Check sheet for the drawn part. Datum: minimum x, y, z corner. Units: mm. Give positions to 0.01 mm unless a question says otherwise; leave off trailing zeros. Write each loop counter-clockwise with the first axis right and the second up, starting at its lowest first coordinate (ties: lowest second). Pieces come first, ordered by that corner, then holes. Notation, with made-up numbers: (27.25, -3.5) - (64.25, -3.5) arc R28 cw to (64.25, 32.5) - close; hole circle Ø9 at (4.25, 85). An arc over 180 degrees is marked (long way). Answer as a JSON object with one key per item and string values. Group by question number.
Item 1: Sectioned sample at B-B, the plane x = 5. Record the boundary of the cut face in (y, z).
Item 2: Scan lines: line 1 along Y through (x, z) = (5, 1.2); line 2 along X through (y, z) = (25, 1.5); line 3 along Y through (x, z) = (7, 1.7). Record each from-to range of solid material in increasing order. Write a range as [from, to].
Item 3: Sectioned sample at C-C, the plane z = 1.55. Record the boundary of the cut face in (x, y).
Item 4: Sectioned sample at A-A, the plane y = 5. Record the boundary of the cut face in (x, z), and give its area (3 significant figures).
Item 5: Draft check along X on the marked faces 1, 2, 3 and 4. Enter one of: +X half, -X half, draft (parallel to the pull), parting line (faces both ways), or undercut.
Item 6: Sectioned sample at D-D, the plane x = 3.25. Record the boundary of the cut face in (y, z).
Item 7: Go/stop test with flat-tipped pins: pin 1 (2 mm diameter, centred on x = 8, y = 10.5, fed in from -Z); pin 2 (5.5 mm diameter, centred on x = 5, y = 25, fed in from -Z). Record where each tip stops, or that it passes through.
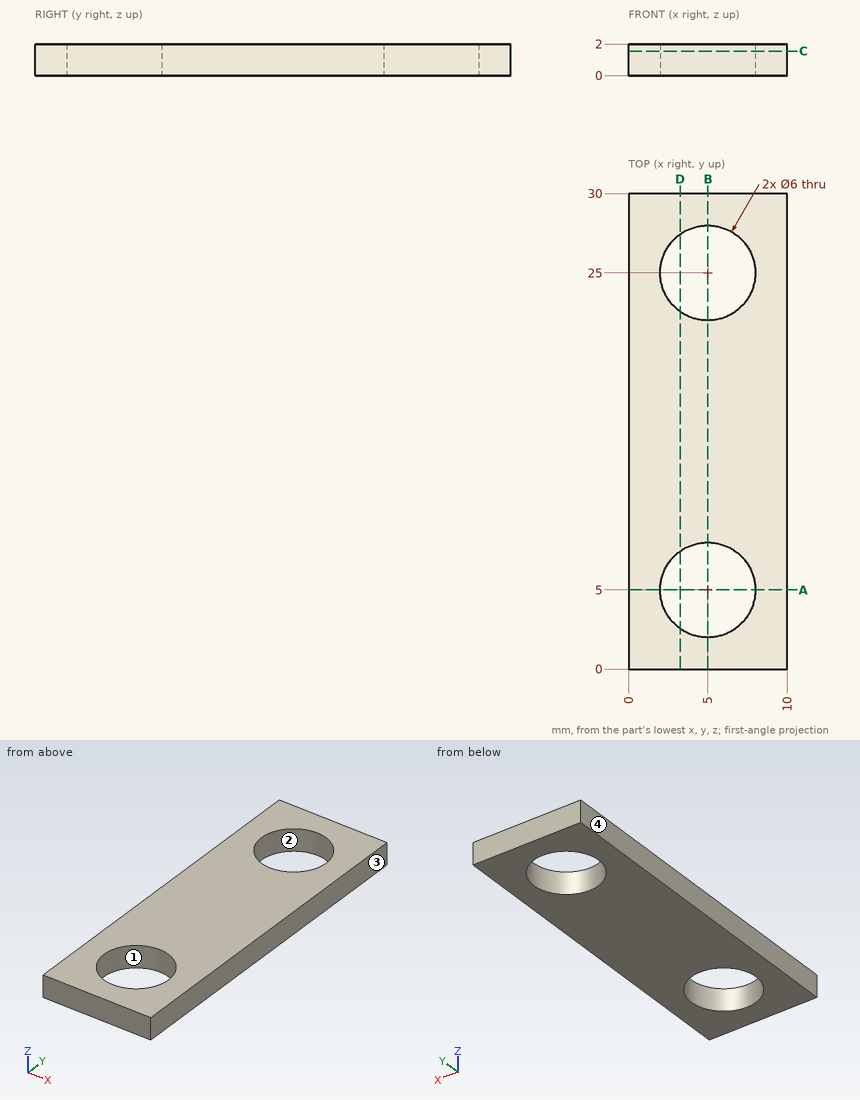
Geometry check:
{
 "1": {"outline": "(0, 0) - (2, 0) - (2, 2) - (0, 2) - close; (8, 0) - (22, 0) - (22, 2) - (8, 2) - close; (28, 0) - (30, 0) - (30, 2) - (28, 2) - close"},
 "2": {"line 1": "[0, 2], [8, 22], [28, 30]", "line 2": "[0, 2], [8, 10]", "line 3": "[0, 2.76], [7.24, 22.76], [27.24, 30]"},
 "3": {"outline": "(0, 0) - (10, 0) - (10, 30) - (0, 30) - close; hole circle Ø6 at (5, 5); hole circle Ø6 at (5, 25)"},
 "4": {"outline": "(0, 0) - (2, 0) - (2, 2) - (0, 2) - close; (8, 0) - (10, 0) - (10, 2) - (8, 2) - close", "area": "8.00 mm^2"},
 "5": {"face 1": "undercut", "face 2": "undercut", "face 3": "+X half", "face 4": "-X half"},
 "6": {"outline": "(0, 0) - (2.56, 0) - (2.56, 2) - (0, 2) - close; (7.44, 0) - (22.56, 0) - (22.56, 2) - (7.44, 2) - close; (27.44, 0) - (30, 0) - (30, 2) - (27.44, 2) - close"},
 "7": {"pin 1": "z = 0", "pin 2": "through"}
}
